```python
from build123d import *

# Parameters (mm, degrees)
F0_W     = 102.7684
F0_H     = 101.6
F1_DEPTH = 101.6
F2_R     = 25.4
F3_DEPTH = 101.6
F6_W     = 50.8
F6_H     = 50.8
F7_DEPTH = 101.6
F8_R     = 6.35
F9_R     = 5.08


with BuildPart() as f1:
    # F0 (on Top) → F1 (new body)
    with BuildSketch(Plane.XY):
        with Locations((2.4761343375, 0)):
            Rectangle(F0_W, F0_H)
    extrude(amount=F1_DEPTH)

    # F2 (on face) → F3 (join)
    with BuildSketch(Plane.XY.offset(101.6)):
        Circle(F2_R)
    extrude(amount=F3_DEPTH)

    # F4 (on face) → F5 (revolve)
    with BuildSketch(Plane.XY.offset(203.2)):
        with BuildLine():
            ThreePointArc((0, -38.1876719344), (27.0027617826, -27.0027617826), (38.1876719344, 0))
            ThreePointArc((38.1876719344, 0), (27.0027617826, 27.0027617826), (0, 38.1876719344))
            Line((0, 38.1876719344), (0, 25.4))
            ThreePointArc((0, 25.4), (17.9605122421, 17.9605122421), (25.4, 0))
            ThreePointArc((25.4, 0), (17.9605122421, -17.9605122421), (0, -25.4))
            Line((0, -25.4), (0, -38.1876719344))
        make_face()
    revolve(axis=Axis((0, -1.256869865, 203.2), (0, -1, 0)))

    # F6 (on face) → F7 (cut)
    with BuildSketch(Plane.XZ.offset(50.8)):
        with Locations((0, 43.5710921884)):
            Rectangle(F6_W, F6_H)
    extrude(amount=-F7_DEPTH, mode=Mode.SUBTRACT)

    # F8
    f8_edges = [f1.edges().sort_by_distance(p)[0] for p in [
        (53.860334, 0, 101.6),
        (53.860334, -50.8, 50.8),
        (53.860334, 50.8, 50.8),
        (53.860334, 0, 0),
        (2.476134, -50.8, 101.6),
        (-48.908066, -50.8, 50.8),
        (-48.908066, 0, 101.6),
        (2.476134, 50.8, 101.6),
        (2.476134, -50.8, 0),
        (-48.908066, 0, 0),
        (2.476134, 50.8, 0),
    ]]
    fillet(f8_edges, radius=F8_R)

    # F9
    f9_edges = [f1.edges().sort_by_distance(p)[0] for p in [
        (-25.4, 0, 101.6),
        (-25.4, 0, 174.68442),
    ]]
    fillet(f9_edges, radius=F9_R)


solid = f1.part
```
The listing builds one solid part. Answer for the finished solid, in the listing's coordinates (mm). A direction names the side the tool comes from. Give positions to 0.01 mm unless a question says otherwise; leave off trailing zeros. Loops run counter-clockwise (first coordinate to the right, second up) from the corner with the lowest first, then second, coordinate; pieces in that order, holes last. Notation, with made-up numbers: (65, 78.25) - (116, 78.25) arc R26 ccw to (116, 110.25) - close; hole circle Ø8 at (38, 0.25). An arc over 180 degrees is marked (long way). Return JSON: item names as keys, results as strings. Group by question number.
1. Given pin 1 Ø1.5 at (y, z) = (-9, 124) entering from -X; pin 2 Ø1 at (y, z) = (-1.5, 164.5) entering from +X; pin 3 Ø5 at (y, z) = (19.5, 177.5) entering from +X, each flat-ended and moving along its own axis, determine where each tip first touches the part or whether it passes through.
2. Determine the mould class of faces 4 (the cylindrical face through (-47, 3.84, 99.79)), 5 (the cylindrical face through (-0.02, 48.89, 99.79)), 6 (the flat face through (0, 0, 203.2)) for opening direction X: pulls with the +X half, pulls with the -X half, needs draft (parallel to the pull), parting line crosses it, or undercut.
3. Find section C-C (x = 42). Write down the section's boundary in (y, z), then the cut area to 3 significant figures.
4. Which of the six approach directions +Z, -Z, +X, -X, +Y, -Y give full straight-line access (tool end or side, diameter ignored) to faces 1 (the flat face through (-48.908, 3, 50)), 2 (the flat face through (25.4, -1, 43)), 3 (the flat face through (32, 1, 101.6))?
5. Find section A-A (z = 36). Write down the section's boundary in (x, y), then the cut area to 3 significant figures.
6. Straight lines are drawn through the part: line 1 (X direction, y = 45, z = 59); line 2 (Z direction, x = -14.5, y = -36.5); line 3 (Z direction, x = -14, y = 8). For each, find the intervals that lie inside material, in ascending order. Write a range as [from, to].
7. Find section B-B (x = 0). State how many separate pieces and enclosed holes the cut face has, then the cut area to 3 significant figures.
Verdict:
{
 "1": {"pin 1": "stops at x = -24.02", "pin 2": "stops at x = 25.38", "pin 3": "stops at x = 23.93"},
 "2": {"face 4": "pulls with the -X half", "face 5": "needs draft", "face 6": "undercut"},
 "3": {"outline": "(-50.8, 6.35) arc R6.35 ccw to (-44.45, 0) - (44.45, 0) arc R6.35 ccw to (50.8, 6.35) - (50.8, 95.25) arc R6.35 ccw to (44.45, 101.6) - (-44.45, 101.6) arc R6.35 ccw to (-50.8, 95.25) - close", "area": "10,300 mm^2"},
 "4": {"face 1": "+Z, -Z, -X, +Y, -Y", "face 2": "+Y, -Y", "face 3": "none"},
 "5": {"outline": "(-48.91, -44.45) arc R6.35 ccw to (-42.56, -50.8) - (-25.4, -50.8) - (-25.4, 50.8) - (-48.91, 50.8) - close; (25.4, -50.8) - (47.51, -50.8) arc R6.35 ccw to (53.86, -44.45) - (53.86, 44.45) arc R6.35 ccw to (47.51, 50.8) - (25.4, 50.8) - close", "area": "5,250 mm^2"},
 "6": {"line 1": "x = [-48.91, -25.4], [25.4, 53.84]", "line 2": "z = [0, 18.17], [68.97, 101.6]", "line 3": "z = [0, 18.17], [68.97, 203.2], [222.83, 237.82]"},
 "7": {"separate pieces": "2", "enclosed holes": "1", "area": "12,100 mm^2"}
}
